```python
from build123d import *

# Parameters (mm, degrees)
SKETCH1_W               = 45
SKETCH1_H               = 20
BOSS_EXTRUDE1_DEPTH     = 3
CUT_EXTRUDE1_DEPTH      = 25.80423351
CUT_EXTRUDE1_DEPTH_BACK = 25.80423351
SKETCH2_R               = 8.25
SKETCH2_R_2             = 0.75
BOSS_EXTRUDE2_DEPTH     = 3
BOSS_EXTRUDE3_DEPTH     = 3
SKETCH9_W               = 10
SKETCH9_H               = 4
BOSS_EXTRUDE4_DEPTH     = 30
CUT_EXTRUDE2_DEPTH      = 3
CUT_EXTRUDE3_DEPTH      = 56.563027275
CUT_EXTRUDE3_DEPTH_BACK = 56.563027275
SKETCH11_R              = 0.625
SKETCH11_R_2            = 1.5
CUT_EXTRUDE4_DEPTH      = 48.11952886
CUT_EXTRUDE4_DEPTH_BACK = 48.11952886
SKETCH12_W              = 12
SKETCH12_H              = 3


with BuildPart() as part:
    # Sketch1 → Boss-Extrude1 (new body)
    with BuildSketch(Plane.XY):
        Rectangle(SKETCH1_W, SKETCH1_H)
    extrude(amount=BOSS_EXTRUDE1_DEPTH)

    # Sketch2 → Cut-Extrude1 (cut, two sides: drawn at the far end of the back side and taken through both)
    with BuildSketch(Plane.XY.offset(3).offset(-CUT_EXTRUDE1_DEPTH_BACK)):
        with Locations((-13.5, 0)):
            Circle(SKETCH2_R)
        with Locations(Location((13.5, 0, 0), (0, 0, 180))):
            Circle(SKETCH2_R)
        with Locations((-21.5, -9)):
            Circle(SKETCH2_R_2)
        with Locations((21.5, 9)):
            Circle(SKETCH2_R_2)
    extrude(amount=CUT_EXTRUDE1_DEPTH + CUT_EXTRUDE1_DEPTH_BACK, mode=Mode.SUBTRACT)

    # Sketch7 → Boss-Extrude2 (add)
    with BuildSketch(Plane.XY.offset(3)):
        Polygon((-15, 25), (-22.5, 10), (-7.5, 10), align=None)
        Polygon((15, 25), (7.5, 10), (22.5, 10), align=None)
    extrude(amount=-BOSS_EXTRUDE2_DEPTH)

    # Sketch8 → Boss-Extrude3 (add)
    with BuildSketch(Plane.XY.offset(3)):
        Polygon((-5, -13), (-5, -20), (5, -20), (5, -13), (9, -13), (9, -10), (-9, -10), (-9, -13), align=None)
    extrude(amount=-BOSS_EXTRUDE3_DEPTH)

    # Sketch9 → Boss-Extrude4 (add)
    with BuildSketch(Plane(origin=(0, 0, 0), x_dir=(-1, 0, 0), z_dir=(0, 0, -1))):
        with Locations((0, -18)):
            Rectangle(SKETCH9_W, SKETCH9_H)
    extrude(amount=BOSS_EXTRUDE4_DEPTH)

    # Sketch10 → Cut-Extrude2 (cut)
    with BuildSketch(Plane.XZ.offset(20)):
        with BuildLine():
            Line((-4, -11), (-3, -24))
            ThreePointArc((-3, -24), (0, -27), (3, -24))
            Line((3, -24), (4, -11))
            ThreePointArc((4, -11), (0, -7), (-4, -11))
        make_face()
    extrude(amount=-CUT_EXTRUDE2_DEPTH, mode=Mode.SUBTRACT)

    # Sketch11 → Cut-Extrude3 (cut, two sides: drawn at the far end of the back side and taken through both)
    with BuildSketch(Plane(origin=(0, -16, 0), x_dir=(1, 0, 0), z_dir=(0, 1, 0)).offset(-CUT_EXTRUDE3_DEPTH_BACK)):
        with Locations(Location((0, 15.5, 0), (0, 0, 90))):
            Circle(SKETCH11_R)
        with Locations(Location((0, 19.5, 0), (0, 0, 90))):
            Circle(SKETCH11_R)
        with Locations(Location((0, 11, 0), (0, 0, 90))):
            Circle(SKETCH11_R_2)
        with Locations(Location((0, 23.5, 0), (0, 0, 90))):
            Circle(SKETCH11_R)
    extrude(amount=CUT_EXTRUDE3_DEPTH + CUT_EXTRUDE3_DEPTH_BACK, mode=Mode.SUBTRACT)

    # Sketch12 → Cut-Extrude4 (cut, two sides: drawn at the far end of the back side and taken through both)
    with BuildSketch(Plane.XY.offset(3).offset(-CUT_EXTRUDE4_DEPTH_BACK)):
        with BuildLine():
            Line((-3.3, -5.25), (3.3, -5.25))
            ThreePointArc((3.3, -5.25), (5.55, -7.5), (3.3, -9.75))
            Line((3.3, -9.75), (-3.3, -9.75))
            ThreePointArc((-3.3, -9.75), (-5.55, -7.5), (-3.3, -5.25))
        make_face()
        with Locations((0, 8.5)):
            Rectangle(SKETCH12_W, SKETCH12_H)
    extrude(amount=CUT_EXTRUDE4_DEPTH + CUT_EXTRUDE4_DEPTH_BACK, mode=Mode.SUBTRACT)


solid = part.part
```
CAD build for the part. Positions are in the model's coordinates, mm. A direction names the side the tool comes from. Coordinates: 2 decimals unless noted, no trailing zeros. Write each loop counter-clockwise with the first axis right and the second up, starting at its lowest first coordinate (ties: lowest second). Pieces come first, ordered by that corner, then holes. Notation, with made-up numbers: (62, -12) -> (114, -12) arc R23 cw to (114, 18) -> close; hole circle Ø7 at (27.5, -12). An arc over 180 degrees is marked (long way). Return JSON: item names as keys, results as strings. Group by question number.
Q1. Cut at C-C, the plane y = 9. Give the cut face in (x, z), then the cut area to 3 significant figures.
Q2. Cut at B-B, the plane x = 0. State how many separate pieces and enclosed holes the cut face has, then the cut area to 3 significant figures.
Q3. Pull direction X, two halves, no side cores. Call faces 1 (the face through (0, 5, 0)), 2 (the face through (6, 8, 1)), 3 (the face through (-9, -11, 2)), 4 (the face through (19, 17, 2)): released by +X, released by -X, zero draft, split by the parting line, or undercut.
Q4. Cut at A-A, the plane y = 22. Give the cut face in (x, z).
Q5. Drill centre lines: line 1 (X direction, y = 9, z = 2); line 2 (X direction, y = -15, z = 1.5); line 3 (Z direction, x = -10.5, y = 12). Where is each one in solid material? Low to high.
Q6. Flat gauge pins, fed straight in: pin 1 (2.5 mm diameter, centred on x = -1, z = 1, fed in from +Y); pin 2 (0.8 mm diameter, centred on x = 0, z = -23.5, fed in from -Y); pin 3 (6 mm diameter, centred on y = -14.5, z = -24, fed in from -X); pin 4 (3.5 mm diameter, centred on x = 16, z = 1, fed in from -Y). Where does each tip first touch, or does it go through?
Q7. Cut at D-D, the plane z = -15.5. Give the cut face in (x, y) (3 decimals), then the cut area to 3 significant figures.
Q8. Which spindle directions (+Z, -Z, +X, -X, +Y, -Y) get a long thin tool onto all of the face, cutting with end or side? Do faces 5 (the face through (-6, 8, 1)), 6 (the face through (-5, -18, -13)), 7 (the face through (0, -5.25, 1)), 8 (the face through (-3.507, -18.521, -17.409)). Say none if no direction does.
Returned:
{
 "1": {"outline": "(-22.5, 0) -> (-6, 0) -> (-6, 3) -> (-22.5, 3) -> close; (6, 0) -> (20.75, 0) -> (20.75, 3) -> (6, 3) -> close; (22.25, 0) -> (22.5, 0) -> (22.5, 3) -> (22.25, 3) -> close", "area": "94.5 mm2"},
 "2": {"separate pieces": "6", "enclosed holes": "0", "area": "121 mm2"},
 "3": {"face 1": "zero draft", "face 2": "undercut", "face 3": "released by -X", "face 4": "released by +X"},
 "4": {"outline": "(-16.5, 0) -> (-13.5, 0) -> (-13.5, 3) -> (-16.5, 3) -> close; (13.5, 0) -> (16.5, 0) -> (16.5, 3) -> (13.5, 3) -> close"},
 "5": {"line 1": "x = -22.5 to -6, 6 to 20.75, 22.25 to 22.5", "line 2": "x = -5 to 5", "line 3": "z = 0 to 3"},
 "6": {"pin 1": "stops at y = 7", "pin 2": "passes through", "pin 3": "stops at x = -5", "pin 4": "stops at y = -10"},
 "7": {"outline": "(-5, -20) -> (-3.654, -20) -> (-3.654, -17) -> (-0.625, -17) -> (-0.625, -16) -> (-5, -16) -> close; (0.625, -17) -> (3.654, -17) -> (3.654, -20) -> (5, -20) -> (5, -16) -> (0.625, -16) -> close", "area": "16.8 mm2"},
 "8": {"face 5": "+Z, -Z, +Y", "face 6": "+Z, -Z, -X, -Y", "face 7": "+Z, -Z", "face 8": "-Y"}
}
